Verification items for the finished model (mm, model axes). Round coordinates to 2 decimals unless told otherwise and drop trailing zeros. Write each loop counter-clockwise with the first axis right and the second up, starting at its lowest first coordinate (ties: lowest second). Pieces come first, ordered by that corner, then holes. Notation, with made-up numbers: (84, 80.25) -> (114, 80.25) arc R19 ccw to (114, 86.25) -> close; hole circle Ø7 at (-35, 73). An arc over 180 degrees is marked (long way). Answer as a JSON object with one key per item and string values. Group by question number.
(1) Sectioned sample at A-A on x = 24. Record the cut outline in (y, z).
(2) Scan lines: L1, parallel to X at y = 1.5, z = 5.25; L2, parallel to X at y = 4, z = 4; L3, parallel to Y at x = 26, z = 1.5. Record each from-to range of solid material in increasing order. Write a range as from..to.
(3) Sectioned sample at B-B on x = 9. Record the cut outline in (y, z).
(4) Draft check along X on faces 1 (the face through (0, 3, 4)), 2 (the face through (11, 3.6, 3.5)), 3 (the face through (17, 3, 7)). Enter one of: released by +X, released by -X, zero draft, split by the parting line, or undercut.
```python
from build123d import *

# Parameters (mm, degrees)
SKETCH1_W               = 34
SKETCH1_H               = 7
BOSS_EXTRUDE1_DEPTH     = 7
SKETCH6_OUTSIDE_W       = 43.082
SKETCH6_OUTSIDE_H       = 18.981
SKETCH6_OUTSIDE_W_2     = 34
SKETCH6_OUTSIDE_H_2     = 9.899494937
SKETCH6_OUTSIDE_R       = 2.5
CUT_EXTRUDE2_DEPTH      = 5.949747468
CUT_EXTRUDE2_DEPTH_BACK = 5.949747468


with BuildPart() as part:
    # sketch1 → Boss-Extrude1 (new body)
    with BuildSketch(Plane(origin=(0, 0, 0), x_dir=(1, 0, 0), z_dir=(0, 1, 0))):
        with Locations((17, -3.5)):
            Rectangle(SKETCH1_W, SKETCH1_H)
    extrude(amount=BOSS_EXTRUDE1_DEPTH)

    # Sketch6 outside → Cut-Extrude2 (cut, two sides)
    with BuildSketch(Plane(origin=(0, 0, 0), x_dir=(-1, 0, 0), z_dir=(0, 0.707106781, -0.707106781))) as cut_extrude2_sk:
        with Locations((-17, 4.9495)):
            Rectangle(SKETCH6_OUTSIDE_W, SKETCH6_OUTSIDE_H)
        with Locations((-17, 4.949747469)):
            Rectangle(SKETCH6_OUTSIDE_W_2, SKETCH6_OUTSIDE_H_2, mode=Mode.SUBTRACT)
        with Locations((-25.5, 4.949747468)):
            Circle(SKETCH6_OUTSIDE_R)
        with Locations((-8.5, 4.949747468)):
            Circle(SKETCH6_OUTSIDE_R)
    extrude(amount=CUT_EXTRUDE2_DEPTH, mode=Mode.SUBTRACT)
    extrude(cut_extrude2_sk.sketch, amount=-CUT_EXTRUDE2_DEPTH_BACK, mode=Mode.SUBTRACT)


solid = part.part
```
Computed values:
{
 "1": {"outline": "(0, 0) -> (4.17, 0) -> (0, 4.17) -> close; (2.83, 7) -> (7, 2.83) -> (7, 7) -> close"},
 "2": {"L1": "0..6.01, 10.99..23.01, 27.99..34", "L2": "0..6.1, 10.9..23.1, 27.9..34", "L3": "0..2.04"},
 "3": {"outline": "(0, 0) -> (3.54, 0) -> (0, 3.54) -> close; (3.46, 7) -> (7, 3.46) -> (7, 7) -> close"},
 "4": {"face 1": "released by -X", "face 2": "undercut", "face 3": "zero draft"}
}
